```python
from build123d import *

# Parameters (mm, degrees)
BOSS_EXTRUDE1_DEPTH = 184.3
CUT_EXTRUDE3_DEPTH  = 38.907676661
SKETCH5_W           = 20
SKETCH5_H           = 5
SKETCH5_W_2         = 3
SKETCH5_H_2         = 20
SKETCH5_H_3         = 3
BOSS_EXTRUDE2_DEPTH = 5


with BuildPart() as part:
    # Sketch2 → Boss-Extrude1 (new body)
    with BuildSketch(Plane.XY.offset(34.9)):
        Polygon((-52.961538618, -36.862052104), (-51.252736373, -41.56098761), (-147.541457764, -76.577085001), (-149.250260009, -71.878149495), align=None)
    extrude(amount=BOSS_EXTRUDE1_DEPTH)

    # Sketch4 → Cut-Extrude3 (cut, through all)
    with BuildSketch(Plane(origin=(7.362313595, -20.245196221, 0), x_dir=(-0.939787101, -0.341760449, 0), z_dir=(0.341760449, -0.939787101, 0))):
        Polygon((111.499570088, -34.9), (115.699570088, -34.9), (115.699570088, -38.9), (117.399570088, -38.9), (117.399570088, -41.7), (115.699570088, -41.7), (115.699570088, -51.7), (111.499570088, -51.7), (111.499570088, -41.7), (109.799570088, -41.7), (109.799570088, -38.9), (111.499570088, -38.9), align=None)
        Polygon((62.37056233, -83.075), (62.37056233, -78.875), (66.37056233, -78.875), (66.37056233, -77.175), (69.17056233, -77.175), (69.17056233, -78.875), (79.17056233, -78.875), (79.17056233, -83.075), (69.17056233, -83.075), (69.17056233, -84.775), (66.37056233, -84.775), (66.37056233, -83.075), align=None)
        Polygon((115.699570088, -219.2), (111.499570088, -219.2), (111.499570088, -215.2), (109.799570088, -215.2), (109.799570088, -212.4), (111.499570088, -212.4), (111.499570088, -202.4), (115.699570088, -202.4), (115.699570088, -212.4), (117.399570088, -212.4), (117.399570088, -215.2), (115.699570088, -215.2), align=None)
        Polygon((66.37056233, -175.225), (66.37056233, -176.925), (69.17056233, -176.925), (69.17056233, -175.225), (79.17056233, -175.225), (79.17056233, -171.025), (69.17056233, -171.025), (69.17056233, -169.325), (66.37056233, -169.325), (66.37056233, -171.025), (62.37056233, -171.025), (62.37056233, -175.225), align=None)
        Polygon((164.828577846, -171.025), (164.828577846, -175.225), (160.828577846, -175.225), (160.828577846, -176.925), (158.028577846, -176.925), (158.028577846, -175.225), (148.028577846, -175.225), (148.028577846, -171.025), (158.028577846, -171.025), (158.028577846, -169.325), (160.828577846, -169.325), (160.828577846, -171.025), align=None)
        Polygon((160.828577846, -78.875), (160.828577846, -77.175), (158.028577846, -77.175), (158.028577846, -78.875), (148.028577846, -78.875), (148.028577846, -83.075), (158.028577846, -83.075), (158.028577846, -84.775), (160.828577846, -84.775), (160.828577846, -83.075), (164.828577846, -83.075), (164.828577846, -78.875), align=None)
    extrude(amount=-CUT_EXTRUDE3_DEPTH, mode=Mode.SUBTRACT)

    # Sketch5 → Boss-Extrude2 (add)
    with BuildSketch(Plane(origin=(7.362313595, -20.245196221, 0), x_dir=(0.939787101, 0.341760449, 0), z_dir=(0.341760449, -0.939787101, 0))):
        with Locations((-86.935066209, 32.4)):
            Rectangle(SKETCH5_W, SKETCH5_H)
        with Locations((-140.264073967, 32.4)):
            Rectangle(SKETCH5_W, SKETCH5_H)
        with Locations((-60.87056233, 127.05)):
            Rectangle(SKETCH5_W_2, SKETCH5_H_2)
        with Locations((-60.87056233, 197.2125)):
            Rectangle(SKETCH5_W_2, SKETCH5_H_2)
        with Locations((-86.935066209, 220.7)):
            Rectangle(SKETCH5_W, SKETCH5_H_3)
        with Locations((-140.264073967, 220.7)):
            Rectangle(SKETCH5_W, SKETCH5_H_3)
    extrude(amount=-BOSS_EXTRUDE2_DEPTH)


solid = part.part
```
Here's how the part is built. I have some questions about the finished solid (model axes, mm). A direction names the side the tool comes from. Give positions to 0.01 mm unless a question says otherwise; leave off trailing zeros. Loops run counter-clockwise (first coordinate to the right, second up) from the corner with the lowest first, then second, coordinate; pieces in that order, holes last. Notation, with made-up numbers: M -30,25 L 13,25 A19 cw 13,55 Z; hole C -8,2 d11. An arc over 180 degrees is marked long. Return JSON: item names as keys, results as strings.
Item 1: On a 3-axis mill with a long thin cutter (end or side, diameter ignored), from which of +Z, -Z, +X, -X, +Y, -Y can I reach the whole of each face in a straight line? I mean faces 1 (the flat face through (-51, -39, 137.05)), 2 (the flat face through (-132.595, -68.519, 80.946)), 3 (the flat face through (-143, -72, 169.325)). Say none if no direction works.
A:
{"face 1": "+X, +Y", "face 2": "-X, -Y", "face 3": "none"}
Item 2: Imagine slicing it at C-C on x = -112.5. List the corners of the cut face in (y, z) for me.
A:
{"outline": "M -63.83,34.9 L -58.51,34.9 L -58.51,219.2 L -63.83,219.2 Z"}
Item 3: Imagine slicing it at B-B on x = -79.5. List the corners of the cut face in (y, z) for me, then the cut area to 3 significant figures.
A:
{"outline": "M -51.83,29.9 L -46.51,29.9 L -46.51,222.2 L -51.83,222.2 Z", "area": "1,020 mm^2"}
Item 4: Please list where these lines run through material, in increasing order: line 1 (Y direction, x = -65, z = 107); line 2 (Y direction, x = -62, z = 94.5).
A:
{"line 1": "y = -46.56 to -41.24", "line 2": "y = -45.47 to -40.15"}
Item 5: Imagine slicing it at A-A on z = 132.5. List the corners of the cut face in (x, y) for me.
A:
{"outline": "M -149.25,-71.88 L -147.54,-76.58 L -48.43,-40.54 L -50.14,-35.84 Z"}
Item 6: I'm going to push flat-ended pins straight in: pin 1 Ø10 at (x, z) = (-107, 155) entering from -Y; pin 2 Ø12 at (x, y) = (-99, -50) entering from -Z; pin 3 Ø2 at (x, y) = (-100, -58.5) entering from -Z. Where does each tip first touch, or does it pass through?
A:
{"pin 1": "stops at y = -63.65", "pin 2": "stops at z = 34.9", "pin 3": "stops at z = 51.7"}
Item 7: Thinking about a two-plate mould opening in Z: for faces 4 (the flat face through (-132.595, -68.519, 173.154)), 5 (the flat face through (-102.213, -57.47, 217.172)), 6 (the flat face through (-143, -72, 84.775)), 7 (the flat face through (-59, -42, 34.9)), which applies, released by +Z, released by -Z, zero draft, split by the parting line, or undercut?
A:
{"face 4": "undercut", "face 5": "zero draft", "face 6": "undercut", "face 7": "released by -Z"}
